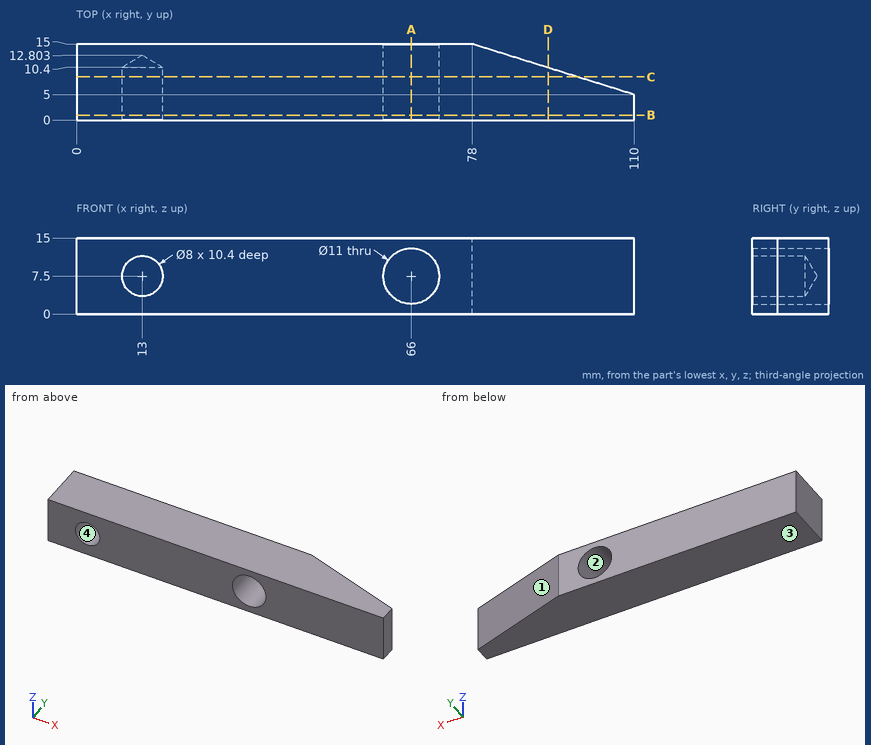
The drawing under review shows one solid part. Ordinate dimensions are in mm from its lowest x, y, z. Give positions to 0.01 mm unless a question says otherwise; leave off trailing zeros. Loops run counter-clockwise (first coordinate to the right, second up) from the corner with the lowest first, then second, coordinate; pieces in that order, holes last. Notation, with made-up numbers: M 18,60.5 L 73,60.5 A17 ccw 73,65.5 Z; hole C -33,62.25 d7. An arc over 180 degrees is marked long. One line per item, written item: value. Start each with the question number.
Q1. Add section B-B (y = 1). Give the boundary of the cut face in (x, z).
Q2. Add section A-A (x = 66). Give the boundary of the cut face in (y, z).
Q3. Draft analysis for pull direction Z (two halves, no side actions). For the marked faces 1, 2, 3 and 4, state which applies: released by +Z, released by -Z, zero draft, split by the parting line, or undercut.
Q4. For L1, parallel to X at y = 2.25, z = 7.5; L2, parallel to Z at x = 13, y = 4.75; L3, parallel to Z at x = 66, y = 10, list the stretches that pass through material, from the lowest coordinate up.
Q5. Add section C-C (y = 8.5). Give the boundary of the cut face in (x, z).
Q6. Add section D-D (x = 93). Give the boundary of the cut face in (y, z), and give its area (3 significant figures).
Q7. Clearance check with flat-ended pins moving along their axes: pin 1 Ø6 at (y, z) = (4.5, 9.5) entering from -X; pin 2 Ø4 at (x, z) = (83, 2) entering from +Y. State where each tip first meets the part, or that it passes through.
Reply:
1. outline: M 0,0 L 110,0 L 110,15 L 0,15 Z; hole C 13,7.5 d8; hole C 66,7.5 d11
2. outline: M 0,0 L 15,0 L 15,2 L 0,2 Z; M 0,13 L 15,13 L 15,15 L 0,15 Z
3. face 1: zero draft
3. face 2: undercut
3. face 3: released by -Z
3. face 4: undercut
4. L1: 0 to 9, 17 to 60.5, 71.5 to 110
4. L2: 0 to 3.5, 11.5 to 15
4. L3: 0 to 2, 13 to 15
5. outline: M 0,0 L 98.8,0 L 98.8,15 L 0,15 Z; hole C 13,7.5 d8; hole C 66,7.5 d11
6. outline: M 0,0 L 10.31,0 L 10.31,15 L 0,15 Z
6. area: 155 mm²
7. pin 1: x = 0
7. pin 2: y = 14.06
